from build123d import *

# Parameters (mm, degrees)
F0_W     = 50.8
F0_H     = 50.8
F0_W_2   = 44.704
F0_H_2   = 44.704
F1_DEPTH = 977.9
F2_R     = 4.7625
F3_DEPTH = 25.4
F4_W     = 50.8
F4_H     = 101.6
F5_DEPTH = 25.4


with BuildPart() as f1:
    # F0 (on Front) → F1 (new body, symmetric)
    with BuildSketch(Plane.XZ):
        with Locations((19.2208130826, 18.3696289983)):
            Rectangle(F0_W, F0_H)
        with Locations((19.2208130826, 18.3696289983)):
            Rectangle(F0_W_2, F0_H_2, mode=Mode.SUBTRACT)
    extrude(amount=F1_DEPTH, both=True)

    # F2 (on face) → F3 (cut)
    with BuildSketch(Plane.XY.offset(-3.9823710017)):
        with Locations((19.2208130826, -965.2)):
            Circle(F2_R)
        with Locations((19.2208130826, -939.8)):
            Circle(F2_R)
        with Locations((19.2208130826, 965.2)):
            Circle(F2_R)
        with Locations((19.2208130826, 939.8)):
            Circle(F2_R)
    extrude(amount=-F3_DEPTH, mode=Mode.SUBTRACT)

    # F4 (on face) → F5 (cut)
    with BuildSketch(Plane.XY.offset(43.7696289983)):
        with Locations((19.2208130826, -977.9)):
            Rectangle(F4_W, F4_H)
        with Locations((19.2208130826, 977.9)):
            Rectangle(F4_W, F4_H)
    extrude(amount=-F5_DEPTH, mode=Mode.SUBTRACT)


solid = f1.part
The listing builds one solid part. Answer for the finished solid, in the listing's coordinates (mm). A direction names the side the tool comes from. Give positions to 0.01 mm unless a question says otherwise; leave off trailing zeros. Loops run counter-clockwise (first coordinate to the right, second up) from the corner with the lowest first, then second, coordinate; pieces in that order, holes last. Notation, with made-up numbers: M -29,29.5 L 30,29.5 A33 ccw 30,61.5 Z; hole C 18,69.5 d1. An arc over 180 degrees is marked long. Answer as CSV lines item,"result".
Item 1: The part is cut by section C-C (y = -563.5). Give the vertices of the cut face in (x, z), and give its area (3 significant figures).
Values follow:
outline,"M -6.18,-7.03 L 44.62,-7.03 L 44.62,43.77 L -6.18,43.77 Z; hole M -3.13,-3.98 L 41.57,-3.98 L 41.57,40.72 L -3.13,40.72 Z"
area,"582 mm^2"
Item 2: Given pin 1 Ø11 at (x, y) = (19.22, 939.8) entering from +Z; pin 2 Ø2.5 at (x, y) = (-4, -944) entering from +Z; pin 3 Ø20.5 at (x, z) = (10, 34) entering from -Y, each flat-ended and moving along its own axis, determine where each tip first touches the part or whether it passes through.
Values follow:
pin 1,"stops at z = -3.98"
pin 2,"stops at z = 18.37"
pin 3,"stops at y = -927.1"
Item 3: Straight lines are drawn through the part: line 1 along Z through (x, y) = (28.5, 147); line 2 along X through (y, z) = (-606, 11); line 3 along X through (y, z) = (939.8, -5.7). For each, find the intervals that lie inside material, in ascending order. Write a range as [from, to].
Values follow:
line 1,"z = [-7.03, -3.98], [40.72, 43.77]"
line 2,"x = [-6.18, -3.13], [41.57, 44.62]"
line 3,"x = [-6.18, 14.46], [23.98, 44.62]"
Item 4: The mould has two halves that part along X. Classify faces 1 (the flat face through (-6.179, -14, 18)), 2 (the flat face through (-3.131, -14, 18)), 3 (the flat face through (19, -13, 43.77)): released by +X, released by -X, zero draft, split by the parting line, or undercut.
Values follow:
face 1,"released by -X"
face 2,"undercut"
face 3,"zero draft"
Item 5: The part is cut by section A-A (z = 31). Give the vertices of the cut face in (x, y), and give its area (3 significant figures).
Values follow:
outline,"M -6.18,-927.1 L -3.13,-927.1 L -3.13,927.1 L -6.18,927.1 Z; M 41.57,-927.1 L 44.62,-927.1 L 44.62,927.1 L 41.57,927.1 Z"
area,"11,300 mm^2"
Item 6: The part is cut by section B-B (x = 5). Give the vertices of the cut face in (y, z).
Values follow:
outline,"M -977.9,-7.03 L 977.9,-7.03 L 977.9,-3.98 L -977.9,-3.98 Z; M -927.1,40.72 L 927.1,40.72 L 927.1,43.77 L -927.1,43.77 Z"
Item 7: Which of the six approach directions +Z, -Z, +X, -X, +Y, -Y give full straight-line access (tool end or side, diameter ignored) to faces 4 (the flat face through (19, -14, -7.03)), 5 (the flat face through (19, -13, 40.722))?
Values follow:
face 4,"-Z, +X, -X, +Y, -Y"
face 5,"+Y, -Y"
